Autodesk Inventor part; units mm, degrees
ref_plane "YZ Plane" through (0, 0, 0) normal (1, 0, 0) x (0, 1, 0)
ref_plane "XZ Plane" through (0, 0, 0) normal (0, 1, 0) x (-1, 0, 0)
ref_plane "XY Plane" through (0, 0, 0) normal (0, 0, 1) x (1, 0, 0)
sketch "スケッチ1" plane through (0, 0, 0) normal (0, 0, 1) x (1, 0, 0)
  line L0 (15, -45.5) -> (-15, -45.5)
  line L1 (-15, -45.5) -> (-15, 45.5)
  line L2 (-15, 45.5) -> (15, 45.5)
  line L3 (15, 45.5) -> (15, -45.5)
  line L4 (15, -45.5) -> (-15, 45.5) construction
  line L5 (-15, -45.5) -> (15, 45.5) construction
  line L6 (-10.25, -20.25) -> (-10.25, 20.25)
  line L7 (-10.25, 20.25) -> (10.25, 20.25)
  line L8 (10.25, 20.25) -> (10.25, -20.25)
  line L9 (10.25, -20.25) -> (-10.25, -20.25)
  line L10 (-10.25, -20.25) -> (10.25, 20.25) construction
  line L11 (-10.25, 20.25) -> (10.25, -20.25) construction
  point P0 (0, 0)
  dimension "d0" = 30
  dimension "d1" = 91
  dimension "d4" = 40.5
  dimension "d5" = 20.5
extrude "押し出し1" add sketch "スケッチ1" along normal blind 40
sketch "スケッチ2" plane through (0, 0, 0) normal (0, 0, -1) x (-1, 0, 0)
  line L0 (-15, -45.5) -> (-15, 45.5)
  line L1 (15, 45.5) -> (15, -45.5)
  line L2 (-15, -45.5) -> (15, -45.5)
  line L3 (15, -45.5) -> (15, -43.5)
  line L4 (15, -43.5) -> (-15, -43.5)
  line L5 (-15, -43.5) -> (-15, -45.5)
  line L6 (-15, 45.5) -> (15, 45.5)
  line L7 (-15, 45.5) -> (15, 45.5)
  line L8 (15, 45.5) -> (15, 43.5)
  line L9 (15, 43.5) -> (-15, 43.5)
  line L10 (-15, 43.5) -> (-15, 45.5)
  point P0 (0, 0)
  point P1 (-15, 43.5)
  dimension "d6" = 2
  dimension "d7" = 2
extrude "押し出し2" add sketch "スケッチ2" along normal blind 50 contours L0 L4 L1 L2 | L0 L6 L1 L9
sketch "スケッチ3" plane through (-15, 45.5, 40) normal (0, 1, 0) x (1, 0, 0)
  line L0 (0, 90) -> (30, 90)
  line L1 (30, 0) -> (30, 90)
  point P0 (15, 40)
  point P1 (15, 86)
  dimension "d10" = 4
  dimension "d11" = 15
hole "穴1" at (0, 45.5, -46) direction (0, -1, 0) diameter 3.2 depth 91
sketch "スケッチ4" plane through (15, -45.5, 40) normal (1, 0, 0) x (0, 0, -1)
  circle A0 centre (27, 55.5) radius 3
  line L0 (0, 0) -> (0, 91)
  line L1 (40, 2) -> (40, 89)
  line L2 (0, 91) -> (90, 91)
  circle A1 centre (14, 55.5) radius 3
  circle A2 centre (27, 35.5) radius 3
  circle A3 centre (14, 35.5) radius 3
  point P0 (40, 45.5)
  point P1 (0, 45.5)
  dimension "d19" = 10
  dimension "d20" = 13
  dimension "d23" = 13
  dimension "d26" = 20
  dimension "d29" = 6
extrude "押し出し3" cut sketch "スケッチ4" against normal up to surface (30 mm away)
properties part number "frame_arm"
Design review of the part built by this model. Coordinates are the model's own, in mm. A direction names the side the tool comes from. Give positions to 0.01 mm unless a question says otherwise; leave off trailing zeros. Order: outer loops, then holes, each group sorted by start corner. A loop starts at its lowest first (then second) coordinate and runs counter-clockwise, first axis right, second up. Notation, with made-up numbers: (13, -9.75) - (63, -9.75) arc R12 cw to (63, 5.25) - close; hole circle Ø4 at (39.5, -38.5). An arc over 180 degrees is marked (long way). Write item = value, one per line. Start each with the question number.
Q1. Clearance check with a flat-ended pin moving along its axis: pin 1 Ø3 at (x, y) = (8, 19) entering from +Z. State where the tip first meets the part, or that it passes through.
Q2. We need section A-A on x = 0. State the section outline as (y, z) points.
Q3. We need section B-B on z = 13. State the section outline as (x, y) points, plus the area to 3 significant figures.
Q4. We need section D-D on x = -7.75. State the section outline as (y, z) points.
Q5. Mouldability with a two-part tool opening along Z and no side actions: class faces 1 (the face through (-14, 1, 0)), 2 (the face through (-13, 10, 29)), 3 (the face through (-10.25, 0, 20)) as released by +Z, released by -Z, zero draft, split by the parting line, or undercut.
Q6. We need section C-C on y = -1. State the section outline as (x, z) points.
Q7. Tool access review of faces 4 (the face through (0, 43.5, -25)), 5 (the face through (13, -10, 29)), 6 (the face through (10.25, 0, 20)): name each direction out of +Z, -Z, +X, -X, +Y, -Y from which nothing blocks a thin tool from reaching the whole face with its end or side.
Q8. To check wall thickness, follow L1, parallel to Y at x = 11.45, z = 26; L2, parallel to Y at x = 13, z = -18; L3, parallel to X at y = 9, z = 1.5. State the ranges of each line that lie inside material, in increasing order. Write a range as from..to.
Working result:
q1.pin_1 = 40
q2.outline = (-45.5, -50) - (-43.5, -50) - (-43.5, -47.6) - (-45.5, -47.6) - close; (-45.5, -44.4) - (-43.5, -44.4) - (-43.5, 0) - (-20.25, 0) - (-20.25, 40) - (-45.5, 40) - close; (20.25, 0) - (43.5, 0) - (43.5, -44.4) - (45.5, -44.4) - (45.5, 40) - (20.25, 40) - close; (43.5, -50) - (45.5, -50) - (45.5, -47.6) - (43.5, -47.6) - close
q3.outline = (-15, -45.5) - (15, -45.5) - (15, -13) - (10.25, -13) - (10.25, -20.25) - (-10.25, -20.25) - (-10.25, -13) - (-15, -13) - close; (-15, -7) - (-10.25, -7) - (-10.25, 7) - (-15, 7) - close; (-15, 13) - (-10.25, 13) - (-10.25, 20.25) - (10.25, 20.25) - (10.25, 13) - (15, 13) - (15, 45.5) - (-15, 45.5) - close; (10.25, -7) - (15, -7) - (15, 7) - (10.25, 7) - close
q3.area = 1,790 mm²
q4.outline = (-45.5, -50) - (-43.5, -50) - (-43.5, 0) - (-20.25, 0) - (-20.25, 40) - (-45.5, 40) - close; (20.25, 0) - (43.5, 0) - (43.5, -50) - (45.5, -50) - (45.5, 40) - (20.25, 40) - close
q5.face_1 = released by -Z
q5.face_2 = undercut
q5.face_3 = zero draft
q6.outline = (-15, 0) - (-10.25, 0) - (-10.25, 40) - (-15, 40) - close; (10.25, 0) - (15, 0) - (15, 40) - (10.25, 40) - close
q7.face_4 = -Z, +X, -X
q7.face_5 = +X, -X
q7.face_6 = +Z, -Z
q8.L1 = -45.5..-13, -7..7, 13..45.5
q8.L2 = -45.5..-43.5, 43.5..45.5
q8.L3 = -15..-10.25, 10.25..15
